```python
from build123d import *

# Parameters (mm, degrees)
BOSS_EXTRUDE1_DEPTH = 50
CUT_EXTRUDE2_DEPTH  = 4
CUT_EXTRUDE14_DEPTH = 6
CUT_EXTRUDE16_DEPTH = 30
HOLE1_D             = 6


with BuildPart() as part:
    # Sketch1 → Boss-Extrude1 (new body)
    with BuildSketch(Plane(origin=(0, 0, 0), x_dir=(1, 0, 0), z_dir=(0, 1, 0))):
        with BuildLine():
            Line((-360, 39.99999406), (360, 39.99999406))
            ThreePointArc((360, 39.99999406), (399.999998105, -4.045e-06), (360, -40))
            Line((360, -40), (-360, -40))
            ThreePointArc((-360, -40), (-399.99999406, -5.94e-06), (-360, 39.99999406))
        make_face()
    extrude(amount=BOSS_EXTRUDE1_DEPTH)

    # Sketch4 → Cut-Extrude2 (cut)
    with BuildSketch(Plane.XZ):
        with BuildLine():
            Line((360, 35.000001075), (-360, 35.000001485))
            ThreePointArc((-360, 35.000001485), (-394.999995545, 5.94e-06), (-360, -34.999989605))
            Line((-360, -34.999989605), (360.000000021, -34.99999406))
            ThreePointArc((360.000000021, -34.99999406), (394.999998105, 4.055e-06), (360, 35.000001075))
        make_face()
    extrude(amount=-CUT_EXTRUDE2_DEPTH, mode=Mode.SUBTRACT)

    # Sketch15 → Cut-Extrude14 (cut)
    with BuildSketch(Plane.XZ.offset(-4)):
        with BuildLine():
            Line((360, -30), (-360, -30))
            ThreePointArc((-360, -30), (-364, -26), (-360, -22))
            Line((-360, -22), (-360, 22))
            ThreePointArc((-360, 22), (-364, 26), (-360, 30))
            Line((-360, 30), (360, 30))
            ThreePointArc((360, 30), (364, 26), (360, 22))
            Line((360, 22), (360, -22))
            ThreePointArc((360, -22), (364, -26), (360, -30))
        make_face()
    extrude(amount=-CUT_EXTRUDE14_DEPTH, mode=Mode.SUBTRACT)

    # Sketch2 → Cut-Extrude16 (cut)
    with BuildSketch(Plane.XZ.offset(-4)):
        with BuildLine():
            Line((356, -26.99999406), (-356, -26.99999406))
            ThreePointArc((-356, -26.99999406), (-358.828427125, -25.828421185), (-360, -22.99999406))
            Line((-360, -22.99999406), (-360, 23))
            ThreePointArc((-360, 23), (-358.828427125, 25.828427125), (-356, 27))
            Line((-356, 27), (356, 27))
            ThreePointArc((356, 27), (358.828427125, 25.828427125), (360, 23))
            Line((360, 23), (360, -22.99999406))
            ThreePointArc((360, -22.99999406), (358.828427125, -25.828421185), (356, -26.99999406))
        make_face()
    extrude(amount=-CUT_EXTRUDE16_DEPTH, mode=Mode.SUBTRACT)

    # Hole1 (through all)
    with Locations(Plane(origin=(0, 4, 0), x_dir=(-1, 0, 0), z_dir=(0, -1, 0))):
        with Locations((-385, 0)):
            Hole(HOLE1_D / 2)


solid = part.part
```
Input: part model. Units: mm. Frame: model coordinates. A direction names the side the tool comes from. Round coordinates to 2 decimals unless told otherwise and drop trailing zeros. Order: outer loops, then holes, each group sorted by start corner. A loop starts at its lowest first (then second) coordinate and runs counter-clockwise, first axis right, second up. Notation, with made-up numbers: (-38, -13) - (21, -13) arc R26 ccw to (21, 8) - close; hole circle Ø6 at (-24.5, 47.5). An arc over 180 degrees is marked (long way). One line per question, with ' | ' between items. Start each with the question number.
1) Set-up query: faces 1 (the flat face through (2, 0, -36)), 2 (the flat face through (-360, 19, 0)). Return all of +Z, -Z, +X, -X, +Y, -Y with unobstructed straight access to the full face (end or side cutting, diameter ignored); none if empty.
2) Contact query for flat-ended pins moving along their axis: P1, Ø15, axis at y = 11.5, z = -4.5, coming from the +X side; P2, Ø3, axis at x = 176.5, z = 12, coming from the -Y side; P3, Ø1.5, axis at y = 27, z = -0.5, coming from the -X side. Output: stop coordinate, or through.
3) Cut plane B-B, the plane x = -169.5. Return the cut outline in (y, z).
4) Pull-direction query (Z, two-part tool) for faces 3 (the flat face through (-5, 22, 27)), 4 (the flat face through (5, 34, 0)), 5 (the flat face through (5, 25, 40)), 6 (the flat face through (6, 50, -1)); classes: +Z half, -Z half, draft (parallel to the pull), parting line (faces both ways), or undercut.
5) Ray query, probe 1 along Z at (x, y) = (240.5, 6); probe 2 along Z at (x, y) = (238, 22.5); probe 3 along Y at (x, z) = (-93.5, -1.5). Return the intervals inside material, ascending.
6) Cut plane A-A, the plane y = 27.5. Return the cut outline in (x, z).
Worked out:
1) face 1: +Z, -Z, +X, -X, -Y | face 2: -Y
2) P1: stops at x = 400 | P2: stops at y = 34 | P3: stops at x = -400
3) outline: (0, -40) - (50, -40) - (50, 40) - (0, 40) - (0, 35) - (4, 35) - (4, 30) - (10, 30) - (10, 27) - (34, 27) - (34, -27) - (10, -27) - (10, -30) - (4, -30) - (4, -35) - (0, -35) - close
4) face 3: undercut | face 4: undercut | face 5: +Z half | face 6: draft
5) probe 1: z = -40 to -30, 30 to 40 | probe 2: z = -40 to -27, 27 to 40 | probe 3: y = 34 to 50
6) outline: (-360, -40) - (360, -40) arc R40 ccw to (360, 40) - (-360, 40) arc R40 ccw to start; hole (-360, -23) arc R4 ccw to (-356, -27) - (356, -27) arc R4 ccw to (360, -23) - (360, 23) arc R4 ccw to (356, 27) - (-356, 27) arc R4 ccw to (-360, 23) - close; hole circle Ø6 at (385, 0)
